Verification items for the finished model (mm, model axes). Give positions to 0.01 mm unless a question says otherwise; leave off trailing zeros. Loops run counter-clockwise (first coordinate to the right, second up) from the corner with the lowest first, then second, coordinate; pieces in that order, holes last. Notation, with made-up numbers: M 15,72.5 L 59,72.5 A35 cw 59,104.5 Z; hole C -39,71 d4. An arc over 180 degrees is marked long. Use CSV: the item, a comma, the result in double quotes.
from build123d import *

# Parameters (mm, degrees)
SKETCH2_W                = 200
SKETCH2_H                = 125
SKETCH2_R                = 1.65
SKETCH2_R_2              = 13
SKETCH2_R_3              = 1.5
SKETCH2_R_4              = 4
BOSS_EXTRUDE1_DEPTH      = 6.35
FILLET1_R                = 50
M6_CLEARANCE_HOLE1_D     = 6.6
M6_CLEARANCE_HOLE1_DEPTH = 15
M6_CLEARANCE_HOLE1_TIP   = 1.982840043


with BuildPart() as part:
    # Sketch2 → Boss-Extrude1 (new body)
    with BuildSketch(Plane(origin=(0, 0, 0), x_dir=(1, 0, 0), z_dir=(0, 1, 0))):
        Rectangle(SKETCH2_W, SKETCH2_H)
        with Locations(Location((-48.5, 0, 0), (0, 0, 270))):
            Circle(SKETCH2_R, mode=Mode.SUBTRACT)
        with Locations(Location((-80.75, -18.619546181, 0), (0, 0, 270))):
            Circle(SKETCH2_R, mode=Mode.SUBTRACT)
        with Locations(Location((-70, 0, 0), (0, 0, 270))):
            Circle(SKETCH2_R_2, mode=Mode.SUBTRACT)
        with Locations(Location((-80.75, 18.619546181, 0), (0, 0, 270))):
            Circle(SKETCH2_R, mode=Mode.SUBTRACT)
        with Locations(Location((-70, 22.5, 0), (0, 0, 270))):
            Circle(SKETCH2_R_3, mode=Mode.SUBTRACT)
        with Locations(Location((43.64387632, 11, 0), (0, 0, 270))):
            Circle(SKETCH2_R_4, mode=Mode.SUBTRACT)
    extrude(amount=BOSS_EXTRUDE1_DEPTH)

    # Fillet1
    fillet1_edges = [part.edges().sort_by_distance(p)[0] for p in [
        (-100, 3.175, 62.5),
        (-100, 3.175, -62.5),
        (100, 3.175, -62.5),
        (100, 3.175, 62.5),
    ]]
    fillet(fillet1_edges, radius=FILLET1_R)

    # M6 Clearance Hole1
    with Locations(Plane(origin=(0, 6.35, 0), x_dir=(1, 0, 0), z_dir=(0, 1, 0))):
        with Locations((60, 50), (-60, -50), (-60, 50), (60, -50)):
            Hole(M6_CLEARANCE_HOLE1_D / 2, depth=M6_CLEARANCE_HOLE1_DEPTH)
            with Locations((0, 0, -(M6_CLEARANCE_HOLE1_DEPTH + M6_CLEARANCE_HOLE1_TIP / 2))):  # 118° drill point
                Cone(0, M6_CLEARANCE_HOLE1_D / 2, M6_CLEARANCE_HOLE1_TIP, mode=Mode.SUBTRACT)


solid = part.part
(1) Scan lines: L1, parallel to X at y = 3, z = 0; L2, parallel to Z at x = 59, y = 1.75; L3, parallel to Z at x = -80.75, y = 2.25. Record each from-to range of solid material in increasing order. Write a range as from..to.
Calculated:
L1,"x = -100..-83, -57..-50.15, -46.85..100"
L2,"z = -61.68..-53.14, -46.86..46.86, 53.14..61.68"
L3,"z = -51.93..-20.27, -16.97..-7.31, 7.31..16.97, 20.27..51.93"
(2) Section check C-C on y = 4.25. Count the separate pieces of the cut face and the enclosed holes in it, plus the area to 3 significant figures.
Calculated:
separate pieces,"1"
enclosed holes,"10"
area,"22,100 mm²"
(3) Section check A-A on z = 6.5. Record the cut outline in (x, y), plus the area to 3 significant figures.
Calculated:
outline,"M -100,0 L -81.26,0 L -81.26,6.35 L -100,6.35 Z; M -58.74,0 L 100,0 L 100,6.35 L -58.74,6.35 Z"
area,"1,130 mm²"
(4) Depth check by flat-ended pin: pin 1 Ø1 at (y, z) = (5, -35.5) entering from +X; pin 2 Ø3 at (y, z) = (4, 18) entering from -X. Enter the tip coordinate at first touch or a pass-through.
Calculated:
pin 1,"stops at x = 94.65"
pin 2,"stops at x = -99.84"
(5) Mould release check, pull along Z, two halves, no side actions. Record for faces 1 (the flat face through (-1, 0, -1)), 2 (the cylindrical face through (-57.11, 3.13, -1.69)), 3 (the flat face through (-1, 3, 62.5)): released by +Z, released by -Z, zero draft, split by the parting line, or undercut.
Calculated:
face 1,"zero draft"
face 2,"undercut"
face 3,"released by +Z"
(6) Section check B-B on x = -61. Record the cut outline in (y, z) (3 decimals).
Calculated:
outline,"M 0,-61.275 L 6.35,-61.275 L 6.35,-53.145 L 0,-53.145 Z; M 0,-46.855 L 6.35,-46.855 L 6.35,-9.381 L 0,-9.381 Z; M 0,9.381 L 6.35,9.381 L 6.35,46.855 L 0,46.855 Z; M 0,53.145 L 6.35,53.145 L 6.35,61.275 L 0,61.275 Z"
(7) Section check D-D on x = 60. Record the cut outline in (y, z).
Calculated:
outline,"M 0,-61.49 L 6.35,-61.49 L 6.35,-53.3 L 0,-53.3 Z; M 0,-46.7 L 6.35,-46.7 L 6.35,46.7 L 0,46.7 Z; M 0,53.3 L 6.35,53.3 L 6.35,61.49 L 0,61.49 Z"
